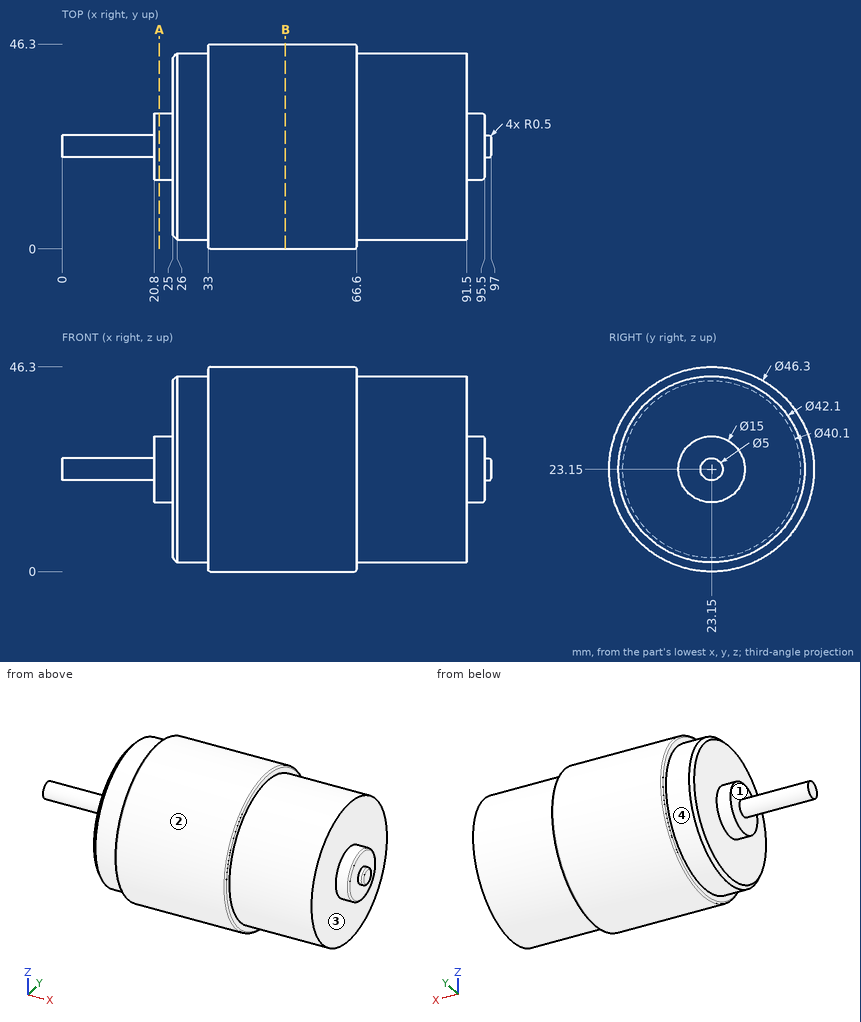
Check sheet for the drawn part. Datum: minimum x, y, z corner. Units: mm. A direction names the side the tool comes from. Give positions to 0.01 mm unless a question says otherwise; leave off trailing zeros. Order: outer loops, then holes, each group sorted by start corner. A loop starts at its lowest first (then second) coordinate and runs counter-clockwise, first axis right, second up.
1. Sectioned sample at A-A (x = 22). Record the boundary of the cut face in (y, z).
Completed:
outline: circle Ø15 at (23.15, 23.15)
2. Access from +Z, -Z, +X, -X, +Y, -Y to the whole of each face (thin tool, end or side, straight path). Record for the marked faces 3 and 4.
Completed:
face 3: +X
face 4: -X
3. Draft check along Y on the marked faces 1 and 2. Enter one of: pulls with the +Y half, pulls with the -Y half, needs draft (parallel to the pull), parting line crosses it, or undercut.
Completed:
face 1: needs draft
face 2: parting line crosses it
4. Sectioned sample at B-B (x = 50.5). Record the boundary of the cut face in (y, z), then the cut area to 3 significant figures.
Completed:
outline: circle Ø46.3 at (23.15, 23.15)
area: 1,680 mm2
5. Scan lines: line 1 (X direction, y = 24.5, z = 13); line 2 (Y direction, x = 38, z = 22.5); line 3 (X direction, y = 37, z = 5.5). Record each from-to range of solid material in increasing order.
Completed:
line 1: x = 25 to 91.5
line 2: y = 0.01 to 46.29
line 3: x = 33 to 66.6
6. Depth check by flat-ended pin: pin 1 (3 mm diameter, centred on x = 63.5, y = 11.5, fed in from +Z); pin 2 (8 mm diameter, centred on x = 31.5, y = 34.5, fed in from -Z) (3 decimals); pin 3 (2 mm diameter, centred on y = 14, z = 33, fed in from -X); pin 4 (4.5 mm diameter, centred on y = 20.5, z = 23.5, fed in from -X). Enter the tip coordinate at first touch or a pass-through.
Completed:
pin 1: stops at z = 43.96
pin 2: stops at z = 1.375
pin 3: stops at x = 25
pin 4: stops at x = 0
